Read the model definition and answer for the solid it produces. Units are mm, in the model's axes. A direction names the side the tool comes from. Coordinates: 2 decimals unless noted, no trailing zeros. Order: outer loops, then holes, each group sorted by start corner. A loop starts at its lowest first (then second) coordinate and runs counter-clockwise, first axis right, second up.
```python
from build123d import *

# Parameters (mm, degrees)
SKETCH2_R           = 31.75
BOSS_EXTRUDE1_DEPTH = 6.35
BOSS_EXTRUDE2_DEPTH = 6.35
SKETCH4_R           = 3.3782
CUT_EXTRUDE1_DEPTH  = 47.6627796
FILLET2_R           = 0.79375
SKETCH5_R           = 2.159
CUT_EXTRUDE2_DEPTH  = 47.6627796
FILLET3_R           = 1.5875


with BuildPart() as part:
    # Sketch2 → Boss-Extrude1 (new body)
    with BuildSketch(Plane.XY):
        Circle(SKETCH2_R)
    extrude(amount=BOSS_EXTRUDE1_DEPTH)

    # Sketch3 → Boss-Extrude2 (add)
    with BuildSketch(Plane.XY.offset(6.35)):
        with BuildLine():
            Line((3.81, 30.613810246), (3.81, 20.6375))
            ThreePointArc((3.81, 20.6375), (0, 16.8275), (-3.81, 20.6375))
            Line((-3.81, 20.6375), (-3.81, 30.613810246))
            ThreePointArc((-3.81, 30.613810246), (-12.7, 21.997045256), (-24.60733738, 18.606461911))
            Line((-24.60733738, 18.606461911), (-15.967599271, 13.618306788))
            ThreePointArc((-15.967599271, 13.618306788), (-14.573042482, 8.41375), (-19.777599271, 7.019193212))
            Line((-19.777599271, 7.019193212), (-28.41733738, 12.007348335))
            ThreePointArc((-28.41733738, 12.007348335), (-25.4, 0), (-28.41733738, -12.007348335))
            Line((-28.41733738, -12.007348335), (-19.777599271, -7.019193212))
            ThreePointArc((-19.777599271, -7.019193212), (-14.573042482, -8.41375), (-15.967599271, -13.618306788))
            Line((-15.967599271, -13.618306788), (-24.60733738, -18.606461911))
            ThreePointArc((-24.60733738, -18.606461911), (-12.7, -21.997045256), (-3.81, -30.613810246))
            Line((-3.81, -30.613810246), (-3.81, -20.6375))
            ThreePointArc((-3.81, -20.6375), (0, -16.8275), (3.81, -20.6375))
            Line((3.81, -20.6375), (3.81, -30.613810246))
            ThreePointArc((3.81, -30.613810246), (12.7, -21.997045256), (24.60733738, -18.606461911))
            Line((24.60733738, -18.606461911), (15.967599271, -13.618306788))
            ThreePointArc((15.967599271, -13.618306788), (14.573042482, -8.41375), (19.777599271, -7.019193212))
            Line((19.777599271, -7.019193212), (28.41733738, -12.007348335))
            ThreePointArc((28.41733738, -12.007348335), (25.4, 0), (28.41733738, 12.007348335))
            Line((28.41733738, 12.007348335), (19.777599271, 7.019193212))
            ThreePointArc((19.777599271, 7.019193212), (14.573042482, 8.41375), (15.967599271, 13.618306788))
            Line((15.967599271, 13.618306788), (24.60733738, 18.606461911))
            ThreePointArc((24.60733738, 18.606461911), (12.7, 21.997045256), (3.81, 30.613810246))
        make_face()
    extrude(amount=BOSS_EXTRUDE2_DEPTH)

    # Sketch4 → Cut-Extrude1 (cut, through all)
    with BuildSketch(Plane.XY.offset(12.7)):
        Circle(SKETCH4_R)
    extrude(amount=-CUT_EXTRUDE1_DEPTH, mode=Mode.SUBTRACT)

    # Fillet2
    fillet2_edges = [part.edges().sort_by_distance(p)[0] for p in [
        (-28.41733738, 12.007348335, 9.525),
        (-28.41733738, -12.007348335, 9.525),
        (-24.60733738, -18.606461911, 9.525),
        (-3.81, -30.613810246, 9.525),
        (3.81, -30.613810246, 9.525),
        (24.60733738, -18.606461911, 9.525),
        (28.41733738, -12.007348335, 9.525),
        (28.41733738, 12.007348335, 9.525),
        (24.60733738, 18.606461911, 9.525),
        (3.81, 30.613810246, 9.525),
        (-3.81, 30.613810246, 9.525),
        (-24.60733738, 18.606461911, 9.525),
    ]]
    fillet(fillet2_edges, radius=FILLET2_R)

    # Sketch5 → Cut-Extrude2 (cut, through all)
    with BuildSketch(Plane(origin=(0, 0, 0), x_dir=(-1, 0, 0), z_dir=(0, 0, -1))):
        with Locations((-11.90625, 20.622229928)):
            Circle(SKETCH5_R)
        with Locations((11.90625, 20.622229928)):
            Circle(SKETCH5_R)
        with Locations((23.8125, 0)):
            Circle(SKETCH5_R)
        with Locations((11.90625, -20.622229928)):
            Circle(SKETCH5_R)
        with Locations((-11.90625, -20.622229928)):
            Circle(SKETCH5_R)
        with Locations((-23.8125, 0)):
            Circle(SKETCH5_R)
    extrude(amount=-CUT_EXTRUDE2_DEPTH, mode=Mode.SUBTRACT)

    # Fillet3
    # the kernel refuses this fillet: 1.5875 mm, written as the material it takes off along each edge
    with BuildSketch(Plane(origin=(25.439668824, 1.419014665, 17.971488678), x_dir=(-0.8953649723474578, 0.44533309588805103, 0), z_dir=(0, 0, -1)), Plane(origin=(13.94873716, -21.321892132, 17.971488678), x_dir=(-0.06201271198897514, 0.9980753596556587, 0), z_dir=(0, 0, -1)), Plane(origin=(-11.490931663, -22.740906798, 17.971488678), x_dir=(0.8333522603583458, 0.5527422637682374, 0), z_dir=(0, 0, -1)), Plane(origin=(-25.439668824, -1.419014665, 17.971488678), x_dir=(0.8953649723478783, -0.4453330958872058, 0), z_dir=(0, 0, -1)), Plane(origin=(-13.94873716, 21.321892132, 17.971488678), x_dir=(0.062012711989375524, -0.9980753596556338, 0), z_dir=(0, 0, -1)), Plane(origin=(11.490931663, 22.740906798, 17.971488678), x_dir=(-0.833352260358639, -0.5527422637677954, 0), z_dir=(0, 0, -1))) as fillet3_piece_1:
        with BuildLine():
            CenterArc((2.256551384, 1.467035409), FILLET3_R, 161.515751163, 86.019798363)
            ThreePointArc((0.75094916, 1.970342665), (0.395929534, 0.977375414), (0, 0))
            ThreePointArc((0, 0), (0.824975775, 0.163831844), (1.64995155, 0))
        make_face()
    extrude(amount=11.621488678, mode=Mode.SUBTRACT)
    with BuildSketch(Plane(origin=(25.439668824, -1.419014665, 17.971488678), x_dir=(0.0972615315412338, -0.9952588580275252, 0), z_dir=(0, 0, -1)), Plane(origin=(11.490931663, -22.740906798, 17.971488678), x_dir=(-0.8132886886226869, -0.5818603861394845, 0), z_dir=(0, 0, -1)), Plane(origin=(-13.94873716, -21.321892132, 17.971488678), x_dir=(-0.9105502201639706, 0.4133984718880137, 0), z_dir=(0, 0, -1)), Plane(origin=(-25.439668824, 1.419014665, 17.971488678), x_dir=(-0.09726153154127824, 0.9952588580275209, 0), z_dir=(0, 0, -1)), Plane(origin=(-11.490931663, 22.740906798, 17.971488678), x_dir=(0.8132886886227111, 0.5818603861394509, 0), z_dir=(0, 0, -1)), Plane(origin=(13.94873716, 21.321892132, 17.971488678), x_dir=(0.9105502201639338, -0.41339847188809425, 0), z_dir=(0, 0, -1))) as fillet3_piece_2:
        with BuildLine():
            CenterArc((2.17448908, 1.586131862), FILLET3_R, 181.601297313, 86.019798363)
            ThreePointArc((0.587609026, 1.541770329), (0.446894509, 0.71253856), (0, 0))
            ThreePointArc((0, 0), (1.054297736, 0.021890215), (2.108595471, 0))
        make_face()
    extrude(amount=11.621488678, mode=Mode.SUBTRACT)


solid = part.part
```
1) Flat-ended cylindrical pins translate along their axes: pin 1 Ø6 at (x, z) = (-12.5, 6.5) entering from +Y; pin 2 Ø7 at (y, z) = (23.5, 8) entering from -X; pin 3 Ø1.5 at (y, z) = (21.5, 6) entering from +X; pin 4 Ø4 at (x, y) = (11.91, -20.62) entering from +Z. Find the tip coordinate at first contact, or state that the pin passes through.
A:
pin 1: stops at y = 30.29
pin 2: stops at x = -24.32
pin 3: stops at x = 24.03
pin 4: passes through
2) A cutting plane is placed at C-C, the plane z = 1. Determine the outline of the cut face in (x, y).
A:
outline: circle Ø63.5 at (0, 0); hole circle Ø4.32 at (-23.81, 0); hole circle Ø4.32 at (-11.91, -20.62); hole circle Ø4.32 at (-11.91, 20.62); hole circle Ø6.76 at (0, 0); hole circle Ø4.32 at (11.91, -20.62); hole circle Ø4.32 at (11.91, 20.62); hole circle Ø4.32 at (23.81, 0)
3) Straight lines are drawn through the part: line 1 (Y direction, x = 0, z = 9.5); line 2 (Y direction, x = 22.5, z = 8); line 3 (X direction, y = -7, z = 11). For each, find the intervals that lie inside material, in ascending order.
A:
line 1: y = -16.83 to -3.38, 3.38 to 16.83
line 2: y = -18.64 to -17.4, -8.59 to -1.71, 1.71 to 8.59, 17.4 to 18.64
line 3: x = -26.38 to -19.74, -16 to 16, 19.74 to 26.38
4) A cutting plane is placed at A-A, the plane x = 0. Determine the outline of the cut face in (y, z), and give its area (3 significant figures).
A:
outline: (-31.75, 0) - (-3.38, 0) - (-3.38, 12.7) - (-16.83, 12.7) - (-16.83, 6.35) - (-31.75, 6.35) - close; (3.38, 0) - (31.75, 0) - (31.75, 6.35) - (16.83, 6.35) - (16.83, 12.7) - (3.38, 12.7) - close
area: 531 mm2
5) Which of the six approach directions +Z, -Z, +X, -X, +Y, -Y give full straight-line access (tool end or side, diameter ignored) to faces 5 (the cylindrical face through (14.689, 20.455, 9.569)), 6 (the cylindrical face through (18.893, -19.442, 9.481)), 7 (the cylindrical face through (-18.893, 19.442, 9.481)), 8 (the cylindrical face through (-14.53, 8.49, 9.48)), 9 (the cylindrical face through (4.3, -28.8, 9.6))?
A:
face 5: +Z, +Y
face 6: +Z, +X, -Y
face 7: +Z, -X, +Y
face 8: +Z
face 9: +Z, -Y
6) A cutting plane is placed at D-D, the plane x = 7. Determine the outline of the cut face in (y, z).
A:
outline: (-30.97, 0) - (30.97, 0) - (30.97, 6.35) - (26.48, 6.35) - (26.48, 12.7) - (-26.48, 12.7) - (-26.48, 6.35) - (-30.97, 6.35) - close
7) Determine the mould class of faces 1 (the cylindrical face through (0.08, 16.83, 9.48)), 2 (the flat face through (-23.04, -8.903, 9.481)), 3 (the cylindrical face through (18.98, 19.42, 9.48)), 4 (the cylindrical face through (-26.3, 6.7, 9.5)) for opening direction X: pulls with the +X half, pulls with the -X half, needs draft (parallel to the pull), parting line crosses it, or undercut.
A:
face 1: undercut
face 2: undercut
face 3: pulls with the +X half
face 4: pulls with the -X half
8) A cutting plane is placed at B-B, the plane y = 0. Determine the outline of the cut face in (x, z).
A:
outline: (-31.75, 0) - (-25.97, 0) - (-25.97, 6.35) - (-31.75, 6.35) - close; (-21.65, 0) - (-3.38, 0) - (-3.38, 12.7) - (-21.65, 12.7) - close; (3.38, 0) - (21.65, 0) - (21.65, 12.7) - (3.38, 12.7) - close; (25.97, 0) - (31.75, 0) - (31.75, 6.35) - (25.97, 6.35) - close
